Read the model definition and answer for the solid it produces. Units are mm, in the model's axes. Coordinates: 2 decimals unless noted, no trailing zeros. Order: outer loops, then holes, each group sorted by start corner. A loop starts at its lowest first (then second) coordinate and runs counter-clockwise, first axis right, second up. Notation, with made-up numbers: (22.5, -14.5) -> (38.5, -14.5) arc R14 cw to (38.5, 12.5) -> close; hole circle Ø6 at (-22, -18). An arc over 180 degrees is marked (long way). Answer in a Markdown table with one row per item.
from build123d import *

# Parameters (mm, degrees)
SKETCH3_R           = 2
SKETCH3_R_2         = 5.5
BOSS_EXTRUDE2_DEPTH = 5


with BuildPart() as part:
    # Sketch3 → Boss-Extrude2 (new body)
    with BuildSketch(Plane(origin=(0, 0, 0), x_dir=(1, 0, 0), z_dir=(0, 1, 0))):
        with BuildLine():
            Line((-38.75, 50.75), (28.75, 50.75))
            ThreePointArc((28.75, 50.75), (35.821067812, 47.821067812), (38.75, 40.75))
            Line((38.75, 40.75), (38.75, -40.75))
            ThreePointArc((38.75, -40.75), (35.821067812, -47.821067812), (28.75, -50.75))
            Line((28.75, -50.75), (-38.75, -50.75))
            Line((-38.75, -50.75), (-38.75, 50.75))
        make_face()
        with Locations(Location((-31.75, -43.75, 0), (0, 0, 270))):
            Circle(SKETCH3_R, mode=Mode.SUBTRACT)
        with Locations(Location((-31.75, 43.75, 0), (0, 0, 270))):
            Circle(SKETCH3_R, mode=Mode.SUBTRACT)
        with Locations(Location((31.75, 43.75, 0), (0, 0, 270))):
            Circle(SKETCH3_R, mode=Mode.SUBTRACT)
        with Locations(Location((31.75, -43.75, 0), (0, 0, 270))):
            Circle(SKETCH3_R, mode=Mode.SUBTRACT)
        with Locations(Location((10, -30, 0), (0, 0, 270))):
            Circle(SKETCH3_R_2, mode=Mode.SUBTRACT)
        with BuildLine():
            Line((6.188504231, 32.75), (6.188504231, 27.25))
            ThreePointArc((6.188504231, 27.25), (14.7, 30), (6.188504231, 32.75))
        make_face(mode=Mode.SUBTRACT)
    extrude(amount=BOSS_EXTRUDE2_DEPTH)


solid = part.part
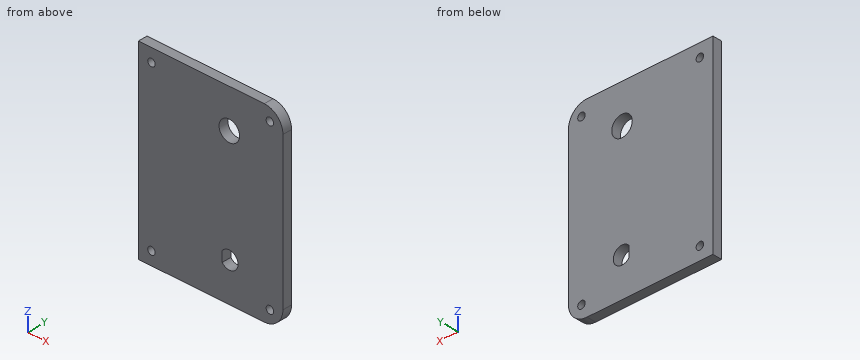
Q1. Consider line 1 (X direction, y = 2.65, z = -43.75); line 2 (X direction, y = 3.4, z = 45.5); line 3 (X direction, y = 2.95, z = -30). Determine where each line is inside the solid, lowest interval first.
Outcome:
| item | result |
|---|---|
| line 1 | -38.75 to -33.75, -29.75 to 29.75, 33.75 to 38.29 |
| line 2 | -38.75 to -32.72, -30.78 to 30.78, 32.72 to 37.55 |
| line 3 | -38.75 to 6.19, 14.7 to 38.75 |
Q2. The part is cut by section D-D (z = -43.75). Write down the section's boundary in (x, y).
Outcome:
| item | result |
|---|---|
| outline | (-38.75, 0) -> (-33.75, 0) -> (-33.75, 5) -> (-38.75, 5) -> close; (-29.75, 0) -> (29.75, 0) -> (29.75, 5) -> (-29.75, 5) -> close; (33.75, 0) -> (38.29, 0) -> (38.29, 5) -> (33.75, 5) -> close |
Q3. The part is cut by section A-A (x = -31.75). Write down the section's boundary in (y, z), then the cut area to 4 significant figures.
Outcome:
| item | result |
|---|---|
| outline | (0, -50.75) -> (5, -50.75) -> (5, -45.75) -> (0, -45.75) -> close; (0, -41.75) -> (5, -41.75) -> (5, 41.75) -> (0, 41.75) -> close; (0, 45.75) -> (5, 45.75) -> (5, 50.75) -> (0, 50.75) -> close |
| area | 467.5 mm² |
Q4. The part is cut by section C-C (y = 3.7). Write down the section's boundary in (x, z).
Outcome:
| item | result |
|---|---|
| outline | (-38.75, -50.75) -> (28.75, -50.75) arc R10 ccw to (38.75, -40.75) -> (38.75, 40.75) arc R10 ccw to (28.75, 50.75) -> (-38.75, 50.75) -> close; hole circle Ø4 at (-31.75, -43.75); hole circle Ø4 at (-31.75, 43.75); hole circle Ø11 at (10, 30); hole (6.19, -32.75) arc R4.7 ccw (long way) to (6.19, -27.25) -> close; hole circle Ø4 at (31.75, -43.75); hole circle Ø4 at (31.75, 43.75) |
Q5. The part is cut by section B-B (z = 30). Write down the section's boundary in (x, y).
Outcome:
| item | result |
|---|---|
| outline | (-38.75, 0) -> (4.5, 0) -> (4.5, 5) -> (-38.75, 5) -> close; (15.5, 0) -> (38.75, 0) -> (38.75, 5) -> (15.5, 5) -> close |
